Read the model definition and answer for the solid it produces. Units are mm, in the model's axes. Face numbers are marked on the shaded views. A direction names the side the tool comes from. Round coordinates to 2 decimals unless told otherwise and drop trailing zeros. Write each loop counter-clockwise with the first axis right and the second up, starting at its lowest first coordinate (ties: lowest second). Pieces come first, ordered by that corner, then holes. Notation, with made-up numbers: (-9.5, 51) - (-3.5, 51) arc R28 cw to (-3.5, 69) - close; hole circle Ø7 at (41, -37.5). An arc over 180 degrees is marked (long way). Use one line per item in the form item = value. Start each with the question number.
1) The part is cut by section C-C, the plane y = 30. Give the vertices of the cut face in (x, z).
2) The part is cut by section D-D, the plane x = 44.5. Give the vertices of the cut face in (y, z).
3) The part is cut by section B-B, the plane z = 6. Give the vertices of the cut face in (x, y), plus the area to 3 significant figures.
4) For the marked faces 1 and 2, determine the directions among +Z, -Z, +X, -X, +Y, -Y from which every point of the face is accessible in a straight line to the end or side of a thin tool.
5) Each of these flat-tipped pins is pushed along its axis until it touches: pin 1 (2 mm diameter, centred on x = 0.5, y = -10.5, fed in from +Z); pin 2 (1.4 mm diameter, centred on x = -11.5, z = 9, fed in from -Y); pin 3 (1.4 mm diameter, centred on y = -11, z = 10, fed in from +X). Where does it stop, or does it pass through?
6) The part is cut by section A-A, the plane x = -51.5. Give the vertices of the cut face in (y, z), plus the area to 3 significant figures.
7) Consider line 1 along Y through (x, z) = (51.5, -0.7); line 2 along X through (y, z) = (0, 3.75); line 3 along X through (y, z) = (0, -1.45). Determine where each line is inside the solid, lowest interval first. Write a range as from..to.
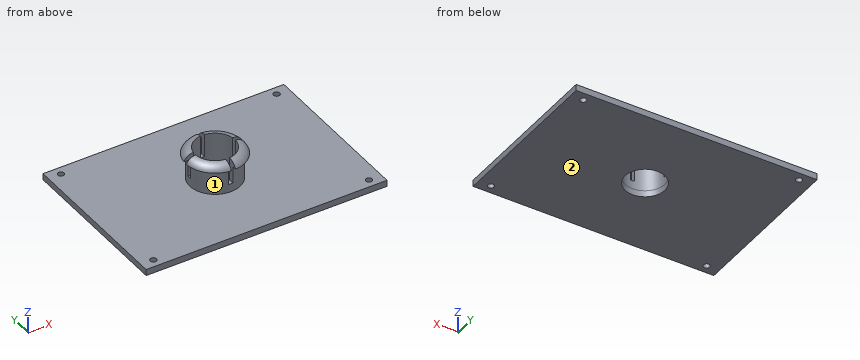
from build123d import *

# Parameters (mm, degrees)
ESBO_O1_R                      = 12
ESBO_O1_R_2                    = 9.5
RESSALTO_EXTRUS_O1_DEPTH       = 12
RESSALTO_EXTRUS_O2_START       = 12
RESSALTO_EXTRUS_O2_OUTLINE_R   = 13.990411925
RESSALTO_EXTRUS_O2_OUTLINE_R_2 = 9.5
RESSALTO_EXTRUS_O2_DEPTH       = 3
CORTE_EXTRUS_O1_DEPTH          = 17
CORTE_EXTRUS_O1_DEPTH_BACK     = 19
ESBO_O2_W                      = 17.351165954
ESBO_O2_H                      = 2
CORTE_EXTRUS_O2_DEPTH          = 19
CORTE_EXTRUS_O2_DEPTH_BACK     = 19
ESBO_O3_W                      = 2
ESBO_O3_H                      = 13.611936421
FILETE1_R                      = 5
FILETE2_R                      = 5
FILETE3_R                      = 5
FILETE4_R                      = 5
RESSALTO_EXTRUS_O3_START       = 3
F_3DSKETCH3_R                  = 9.5
RESSALTO_EXTRUS_O3_DEPTH       = 3
CORTE_EXTRUS_O3_DEPTH          = 14
CORTE_EXTRUS_O3_DEPTH_BACK     = 63
F_3DSKETCH4_R                  = 1.5


with BuildPart() as part:
    # Esboço1 → Ressalto-extrusão1 (new body)
    with BuildSketch(Plane.XY):
        Circle(ESBO_O1_R)
        Circle(ESBO_O1_R_2, mode=Mode.SUBTRACT)
    extrude(amount=RESSALTO_EXTRUS_O1_DEPTH)

    # Ressalto-extrusão2: read off the stored shape, not the designer's step
    # Ressalto-extrusão2 outline → Ressalto-extrusão2 (add)
    with BuildSketch(Plane.XY.offset(RESSALTO_EXTRUS_O2_START)):
        Circle(RESSALTO_EXTRUS_O2_OUTLINE_R)
        Circle(RESSALTO_EXTRUS_O2_OUTLINE_R_2, mode=Mode.SUBTRACT)
    extrude(amount=RESSALTO_EXTRUS_O2_DEPTH)

    # Esboço2 → Corte-extrusão1 (cut, two sides: drawn at the far end of the back side and taken through both)
    with BuildSketch(Plane(origin=(0, 0, 0), x_dir=(0, 0, -1), z_dir=(1, 0, 0)).offset(-CORTE_EXTRUS_O1_DEPTH_BACK)):
        with Locations((-12.675582977, 0.519294875)):
            Rectangle(ESBO_O2_W, ESBO_O2_H)
    extrude(amount=CORTE_EXTRUS_O1_DEPTH + CORTE_EXTRUS_O1_DEPTH_BACK, mode=Mode.SUBTRACT)

    # Esboço3 → Corte-extrusão2 (cut, two sides: drawn at the far end of the back side and taken through both)
    with BuildSketch(Plane(origin=(0, 0, 0), x_dir=(1, 0, 0), z_dir=(0, 1, 0)).offset(-CORTE_EXTRUS_O2_DEPTH_BACK)):
        with Locations((0, -10.80596821)):
            Rectangle(ESBO_O3_W, ESBO_O3_H)
    extrude(amount=CORTE_EXTRUS_O2_DEPTH + CORTE_EXTRUS_O2_DEPTH_BACK, mode=Mode.SUBTRACT)

    # Filete1
    # the kernel refuses this fillet: 5 mm, written as the material it takes off along each edge
    with BuildSketch(Plane(origin=(0, 0, 15), x_dir=(0.7581495843682223, -0.6520806757773855, 0), z_dir=(-0.6520806757773855, -0.7581495843682223, 0))) as filete1_piece_1_section:
        with BuildLine():
            CenterArc((9.40783623, -5), FILETE1_R, 23.578178478, 66.421821522)
            Line((9.40783623, 0), (13.990411925, 0))
            Line((13.990411925, 0), (13.990411925, -3))
        make_face()
    filete1_piece_1 = revolve(axis=Axis((0, 0, 15), (0, 0, 1)), revolution_arc=173.532819647, mode=Mode.PRIVATE)
    filete1_piece_1 = split(filete1_piece_1, bisect_by=Plane(origin=(1, 0, 15), z_dir=(1, 0, 0)), keep=Keep.TOP, mode=Mode.PRIVATE)
    filete1_piece_1 = split(filete1_piece_1, bisect_by=Plane(origin=(0, 1.519294875, 15), z_dir=(0, 1, 0)), keep=Keep.TOP, mode=Mode.PRIVATE)
    add(filete1_piece_1, mode=Mode.SUBTRACT)

    # Filete2
    # the kernel refuses this fillet: 5 mm, written as the material it takes off along each edge
    with BuildSketch(Plane(origin=(0, 0, 15), x_dir=(-0.679899413949249, -0.7333053844828004, 0), z_dir=(-0.7333053844828004, 0.679899413949249, 0))) as filete2_piece_1_section:
        with BuildLine():
            CenterArc((9.40783623, -5), FILETE2_R, 23.578178478, 66.421821522)
            Line((13.990411925, -3), (13.990411925, 0))
            Line((13.990411925, 0), (9.40783623, 0))
        make_face()
    filete2_piece_1 = revolve(axis=Axis((0, 0, 15), (0, 0, 1)), revolution_arc=177.801374174, mode=Mode.PRIVATE)
    filete2_piece_1 = split(filete2_piece_1, bisect_by=Plane(origin=(-1, 0, 15), z_dir=(1, 0, 0)), keep=Keep.TOP, mode=Mode.PRIVATE)
    add(filete2_piece_1, mode=Mode.SUBTRACT)

    # Filete3
    # the kernel refuses this fillet: 5 mm, written as the material it takes off along each edge
    with BuildSketch(Plane(origin=(0, 0, 15), x_dir=(-0.7075313095917145, 0.7066819977524781, 0), z_dir=(0.7066819977524781, 0.7075313095917145, 0))) as filete3_piece_1_section:
        with BuildLine():
            CenterArc((9.40783623, -5), FILETE3_R, 23.578178478, 66.421821522)
            Line((13.990411925, -3), (13.990411925, 0))
            Line((13.990411925, 0), (9.40783623, 0))
        make_face()
    filete3_piece_1 = revolve(axis=Axis((0, 0, 15), (0, 0, 1)), revolution_arc=177.801374174, mode=Mode.PRIVATE)
    filete3_piece_1 = split(filete3_piece_1, bisect_by=Plane(origin=(0, -0.480705125, 15), z_dir=(0, -1, 0)), keep=Keep.TOP, mode=Mode.PRIVATE)
    add(filete3_piece_1, mode=Mode.SUBTRACT)

    # Filete4
    # the kernel refuses this fillet: 5 mm, written as the material it takes off along each edge
    with BuildSketch(Plane(origin=(0, 0, 15), x_dir=(0.6677059228451385, 0.744425147746583, 0), z_dir=(0.744425147746583, -0.6677059228451385, 0))) as filete4_piece_1:
        with BuildLine():
            CenterArc((9.407462566, -4.999143609), FILETE4_R, 23.567471489, 65.372067079)
            Line((13.990411925, -3), (14.082070912, -2.960017128))
            ThreePointArc((14.082070912, -2.960017128), (14.090411925, -1.5), (14.090411925, 0))
            Line((14.090411925, 0), (13.990411925, 0.1))
            ThreePointArc((13.990411925, 0.1), (11.745205963, 0.1), (9.501850749, 0.099982872))
            Line((9.501850749, 0.099982872), (9.5, 0))
        make_face()
    revolve(axis=Axis((0, 0, 15), (0, 0, 1)), revolution_arc=171.645006374, mode=Mode.SUBTRACT)

    # 3DSketch3 → Ressalto-extrusão3 (add)
    with BuildSketch(Plane(origin=(57.5, 39, 0), x_dir=(-0.8275951732462348, -0.5613254218539678, 0), z_dir=(0, 0, -1)).offset(RESSALTO_EXTRUS_O3_START)):
        Polygon((0, 0), (95.173444923, 64.552423513), (138.956827828, 0), (43.783382905, -64.552423513), align=None)
        with Locations(Location((69.478413914, 0, 0), (0, 0, 31.247073166))):
            Circle(F_3DSKETCH3_R, mode=Mode.SUBTRACT)
    extrude(amount=-RESSALTO_EXTRUS_O3_DEPTH)

    # 3DSketch4 → Corte-extrusão3 (cut, two sides: drawn at the far end of the back side and taken through both)
    with BuildSketch(Plane(origin=(51.5, 34.930434783, -3), x_dir=(-0.8275951732462347, -0.5613254218539678, 0), z_dir=(0, 0, 1)).offset(-CORTE_EXTRUS_O3_DEPTH_BACK)):
        with Locations(Location((0, 0, 0), (0, 0, 145.85249086))):
            Circle(F_3DSKETCH4_R)
        with Locations(Location((39.21468208, 57.816518451, 0), (0, 0, 145.85249086))):
            Circle(F_3DSKETCH4_R)
        with Locations(Location((124.456984924, 0, 0), (0, 0, 145.85249086))):
            Circle(F_3DSKETCH4_R)
        with Locations(Location((85.242302844, -57.816518451, 0), (0, 0, 145.85249086))):
            Circle(F_3DSKETCH4_R)
    extrude(amount=CORTE_EXTRUS_O3_DEPTH + CORTE_EXTRUS_O3_DEPTH_BACK, mode=Mode.SUBTRACT)


solid = part.part
Geometry results:
q1.outline = (-57.5, -3) - (57.5, -3) - (57.5, 0) - (-57.5, 0) - close
q2.outline = (-39, -3) - (39, -3) - (39, 0) - (-39, 0) - close
q3.outline = (-11.99, -0.48) arc R12 ccw to (-1, -11.96) - (-1, -9.45) arc R9.5 cw to (-9.49, -0.48) - close; (-11.9, 1.52) - (-9.38, 1.52) arc R9.5 cw to (-1, 9.45) - (-1, 11.96) arc R12 ccw to start; (1, -11.96) arc R12 ccw to (11.99, -0.48) - (9.49, -0.48) arc R9.5 cw to (1, -9.45) - close; (1, 9.45) arc R9.5 cw to (9.38, 1.52) - (11.9, 1.52) arc R12 ccw to (1, 11.96) - close
q3.area = 149 mm2
q4.face_1 = none
q4.face_2 = -Z, +X, -X, +Y, -Y
q5.pin_1 = 14.99
q5.pin_2 = -5.23
q5.pin_3 = 6.16
q6.outline = (-39, -3) - (-36.43, -3) - (-36.43, 0) - (-39, 0) - close; (-33.43, -3) - (33.43, -3) - (33.43, 0) - (-33.43, 0) - close; (36.43, -3) - (39, -3) - (39, 0) - (36.43, 0) - close
q6.area = 216 mm2
q7.line_1 = -39..-36.43, -33.43..33.43, 36.43..39
q7.line_2 = -12..-9.5, 9.5..12
q7.line_3 = -57.5..-9.5, 9.5..57.5
